Check sheet for the drawn part. Datum: minimum x, y, z corner. Units: mm. Coordinates: 2 decimals unless noted, no trailing zeros. Loops run counter-clockwise (first coordinate to the right, second up) from the corner with the lowest first, then second, coordinate; pieces in that order, holes last.
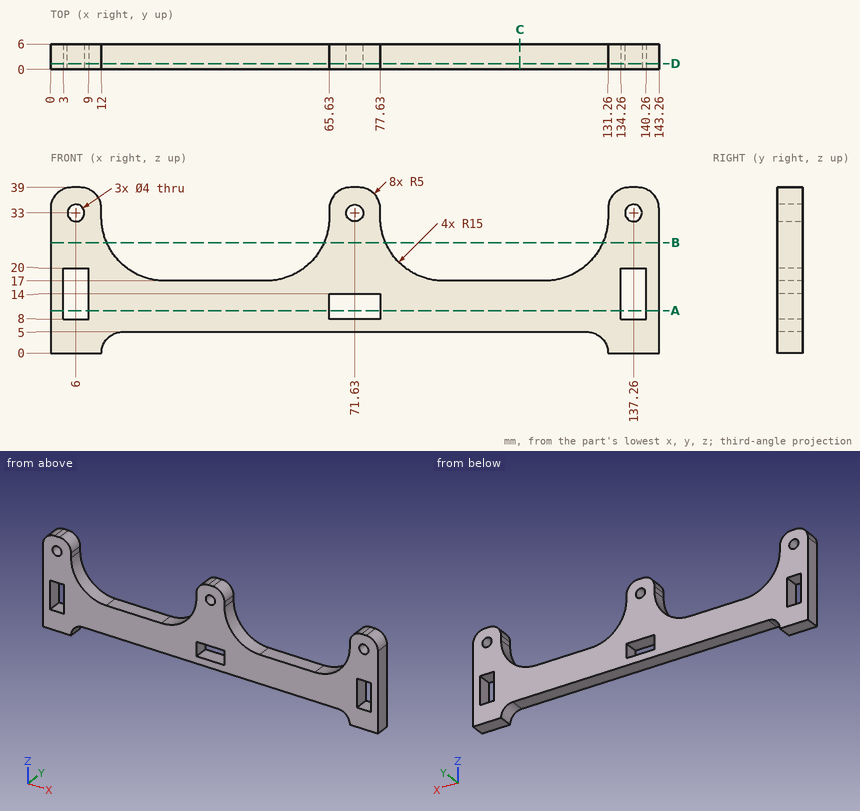
1) Section check B-B on z = 26. Enter the section's corners in (x, y), plus the area to 3 significant figures.
Answer sheet:
outline: (0, 0) - (13.25, 0) - (13.25, 6) - (0, 6) - close; (64.38, 0) - (78.88, 0) - (78.88, 6) - (64.38, 6) - close; (130.01, 0) - (143.26, 0) - (143.26, 6) - (130.01, 6) - close
area: 246 mm2
2) Section check C-C on x = 110.5. Enter the section's corners in (y, z).
Answer sheet:
outline: (0, 5) - (6, 5) - (6, 17) - (0, 17) - close
3) Depth check by flat-ended pin: pin 1 (3 mm diameter, centred on x = 102.5, y = 3.5, fed in from +Z); pin 2 (3 mm diameter, centred on x = 71.63, z = 33, fed in from -Y). Enter the tip coordinate at first touch or a pass-through.
Answer sheet:
pin 1: stops at z = 17
pin 2: passes through
4) Section check A-A on z = 10. Enter the section's corners in (x, y).
Answer sheet:
outline: (0, 0) - (3, 0) - (3, 6) - (0, 6) - close; (9, 0) - (65.63, 0) - (65.63, 6) - (9, 6) - close; (77.63, 0) - (134.26, 0) - (134.26, 6) - (77.63, 6) - close; (140.26, 0) - (143.26, 0) - (143.26, 6) - (140.26, 6) - close
5) Section check D-D on y = 1.35. Give the number of separate pieces and of enclosed holes in the cut face, plus the area to 3 significant figures.
Answer sheet:
separate pieces: 1
enclosed holes: 6
area: 2,550 mm2
6) Scan lines: line 1 (Z direction, x = 137.26, y = 3.55); line 2 (X direction, y = 3.85, z = 18.5); line 3 (Z direction, x = 107, y = 2.85). Record each from-to range of solid material in increasing order.
Answer sheet:
line 1: z = 0 to 8, 20 to 31, 35 to 39
line 2: x = 0 to 3, 9 to 20.46, 57.17 to 86.09, 122.8 to 134.26, 140.26 to 143.26
line 3: z = 5 to 17
